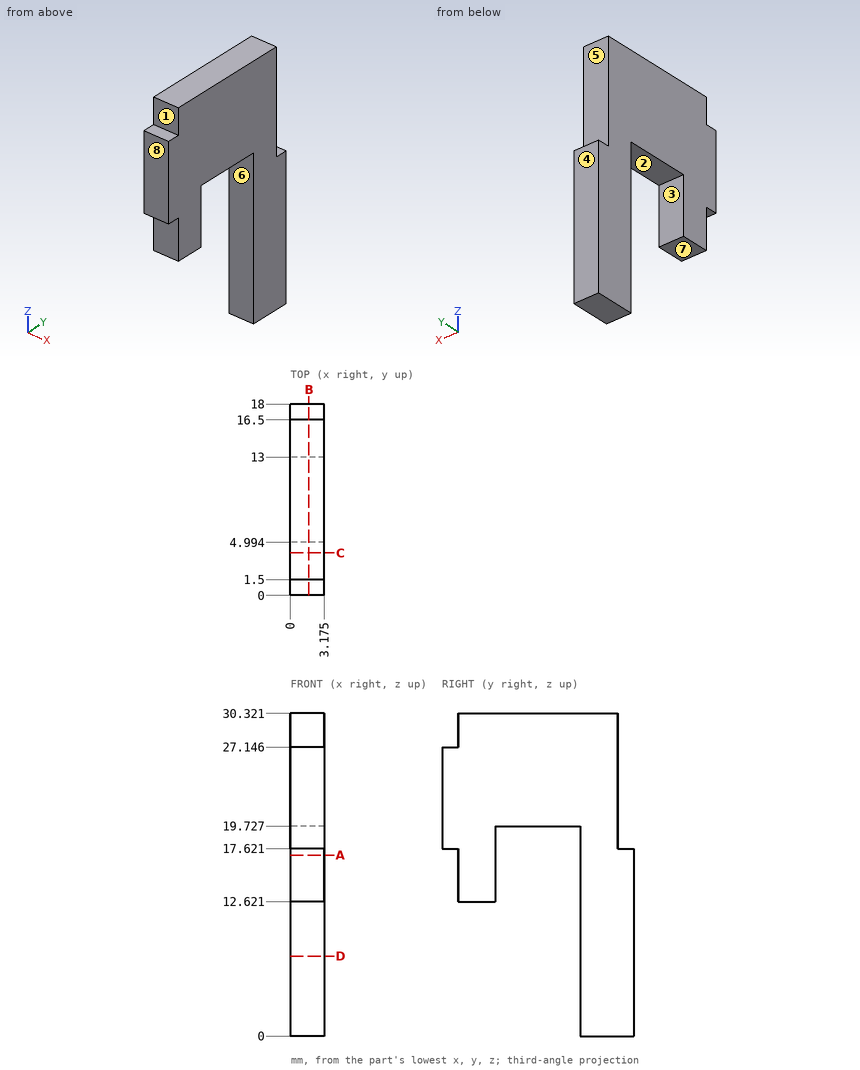
Design review of the part shown in the three views and the two pictorial views. Dimensions are in mm from the part's minimum x, y and z. A direction names the side the tool comes from. Round coordinates to 2 decimals unless told otherwise and drop trailing zeros. Order: outer loops, then holes, each group sorted by start corner. A loop starts at its lowest first (then second) coordinate and runs counter-clockwise, first axis right, second up.
(1) Tool access review of the marked faces 5, 6, 7 and 8: name each direction out of +Z, -Z, +X, -X, +Y, -Y from which nothing blocks a thin tool from reaching the whole face with its end or side.
Working result:
face 5: +Z, +X, -X, +Y
face 6: -Z, +X, -X
face 7: -Z, +X, -X, -Y
face 8: +Z, -Z, +X, -X, -Y
(2) Mouldability with a two-part tool opening along Y and no side actions: class the marked faces 1, 2, 3 and 4 as released by +Y, released by -Y, zero draft, split by the parting line, or undercut.
Working result:
face 1: released by -Y
face 2: undercut
face 3: undercut
face 4: released by +Y
(3) Take a section at D-D, the plane z = 7.5. State the section outline as (x, y) points (1 decimal).
Working result:
outline: (0, 13) - (3.2, 13) - (3.2, 18) - (0, 18) - close
(4) Take a section at C-C, the plane y = 4. State the section outline as (x, z) points (1 decimal), plus the area to 3 significant figures.
Working result:
outline: (0, 12.6) - (3.2, 12.6) - (3.2, 30.3) - (0, 30.3) - close
area: 56.2 mm2
(5) For P1, Ø1, axis at x = 2.5, y = 9, coming from the -Z side; P2, Ø0.8, axis at x = 2.5, y = 0.5, coming from the +Z side; P3, Ø1.6, axis at x = 2, z = 5.5, coming from the -Y side, all flat-tipped, find the tip position at first contact; note any pin that passes through.
Working result:
P1: stops at z = 19.73
P2: stops at z = 27.15
P3: stops at y = 13
(6) Take a section at A-A, the plane z = 17. State the section outline as (x, y) points (1 decimal).
Working result:
outline: (0, 1.5) - (3.2, 1.5) - (3.2, 5) - (0, 5) - close; (0, 13) - (3.2, 13) - (3.2, 18) - (0, 18) - close
(7) Take a section at B-B, the plane x = 1.75. State the section outline as (y, z) points (1 decimal).
Working result:
outline: (0, 17.6) - (1.5, 17.6) - (1.5, 12.6) - (5, 12.6) - (5, 19.7) - (13, 19.7) - (13, 0) - (18, 0) - (18, 17.6) - (16.5, 17.6) - (16.5, 30.3) - (1.5, 30.3) - (1.5, 27.1) - (0, 27.1) - close
(8) Wall thickness on L1, parallel to Y at x = 1.3, z = 18; L2, parallel to Y at x = 1.05, z = 16.5; L3, parallel to Z at x = 0.3, y = 17: over which ranges is each line inside the solid? List them lowest first.
Working result:
L1: y = 0 to 4.99, 13 to 16.5
L2: y = 1.5 to 4.99, 13 to 18
L3: z = 0 to 17.62
